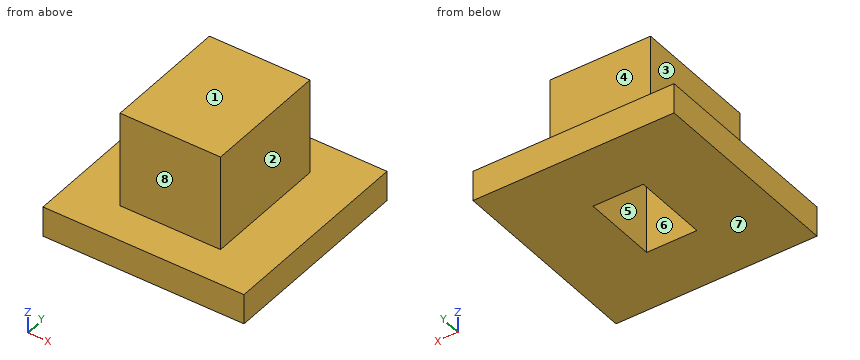
from build123d import *

# Parameters (mm, degrees)
SKETCH_1_W      = 4
SKETCH_1_H      = 5
SKETCH_1_W_2    = 2
SKETCH_1_H_2    = 3
EXTRUDE_1_DEPTH = 4
EXTRUDE_2_DEPTH = 1.2
SKETCH_3_W      = 4
SKETCH_3_H      = 5
EXTRUDE_3_DEPTH = 1
SKETCH_4_W      = 2
SKETCH_4_H      = 8
EXTRUDE_4_DEPTH = 1.2


with BuildPart() as part:
    # 草图1 → 凸台-拉伸1 (new body)
    with BuildSketch(Plane.XY):
        with Locations((1, 1.5)):
            Rectangle(SKETCH_1_W, SKETCH_1_H)
        with Locations((1, 1.5)):
            Rectangle(SKETCH_1_W_2, SKETCH_1_H_2, mode=Mode.SUBTRACT)
    extrude(amount=EXTRUDE_1_DEPTH)

    # 草图2 → 凸台-拉伸2 (add)
    with BuildSketch(Plane(origin=(0, 0, 0), x_dir=(-1, 0, 0), z_dir=(0, 0, -1))):
        Polygon((-3, 4), (1, 4), (1, -1), (-3, -1), (-3, -2.5), (3, -2.5), (3, 5.5), (-3, 5.5), align=None)
    extrude(amount=-EXTRUDE_2_DEPTH)

    # 草图3 → 凸台-拉伸3 (add)
    with BuildSketch(Plane.XY.offset(4)):
        with Locations((1, 1.5)):
            Rectangle(SKETCH_3_W, SKETCH_3_H)
    extrude(amount=EXTRUDE_3_DEPTH)

    # 草图4 → 凸台-拉伸4 (add)
    with BuildSketch(Plane.XY.offset(1.2)):
        with Locations((4, 1.5)):
            Rectangle(SKETCH_4_W, SKETCH_4_H)
    extrude(amount=-EXTRUDE_4_DEPTH)


solid = part.part
CAD build for the part. Positions are in the model's coordinates, mm. Face numbers are marked on the shaded views. A direction names the side the tool comes from. Give positions to 0.01 mm unless a question says otherwise; leave off trailing zeros. Loops run counter-clockwise (first coordinate to the right, second up) from the corner with the lowest first, then second, coordinate; pieces in that order, holes last. Notation, with made-up numbers: M 30.25,76.25 L 85.25,76.25 A30 ccw 85.25,109.25 Z; hole C 87.5,-32.75 d5. An arc over 180 degrees is marked long. Answer in a Markdown table with one row per item. Add a question column.
Item 1: Mould opens along Y. For the marked faces 5, 6, 7 and 8 say: +Y half, -Y half, draft (parallel to the pull), parting line (faces both ways), or undercut.
Item 2: Band-saw the part on D-D on z = 2.8. Give the cut face in (x, y).
Item 3: Drop flat-ended pins along their axis: P1, Ø3, axis at x = -1, z = 4, coming from the +Y side; P2, Ø0.9, axis at y = 1.5, z = 2.5, coming from the -X side; P3, Ø1.9, axis at y = 1, z = 3, coming from the +X side. Give the stop position or say it passes through.
Item 4: Tool access for the marked faces 1, 2, 3 and 4: list every direction of +Z, -Z, +X, -X, +Y, -Y with a clear straight run to the whole face (end or side of a thin tool).
Item 5: Band-saw the part on B-B on y = -0.5. Give the cut face in (x, z).
Item 6: Band-saw the part on A-A on z = 0.8. Give the cut face in (x, y).
Item 7: Probe probe 1 along Y at (x, z) = (0.75, 1.05); probe 2 along X at (y, z) = (0.5, 3.1); probe 3 along Y at (x, z) = (1.25, 2.1). List the from-to ranges inside material, lowest first.
Item 8: Band-saw the part on C-C on x = -0.25. Give the cut face in (y, z), then the cut area to 3 significant figures.
Reply:
| question | item | result |
|---|---|---|
| 1 | face 5 | undercut |
| 1 | face 6 | undercut |
| 1 | face 7 | draft |
| 1 | face 8 | -Y half |
| 2 | outline | M -1,-1 L 3,-1 L 3,4 L -1,4 Z; hole M 0,0 L 2,0 L 2,3 L 0,3 Z |
| 3 | P1 | stops at y = 4 |
| 3 | P2 | stops at x = -1 |
| 3 | P3 | stops at x = 3 |
| 4 | face 1 | +Z, +X, -X, +Y, -Y |
| 4 | face 2 | +Z, +X, +Y, -Y |
| 4 | face 3 | +Z, -X, +Y, -Y |
| 4 | face 4 | +Z, +X, -X, +Y |
| 5 | outline | M -3,0 L 5,0 L 5,1.2 L 3,1.2 L 3,5 L -1,5 L -1,1.2 L -3,1.2 Z |
| 6 | outline | M -3,-2.5 L 5,-2.5 L 5,5.5 L -3,5.5 Z; hole M 0,0 L 2,0 L 2,3 L 0,3 Z |
| 7 | probe 1 | y = -2.5 to 0, 3 to 5.5 |
| 7 | probe 2 | x = -1 to 0, 2 to 3 |
| 7 | probe 3 | y = -1 to 0, 3 to 4 |
| 8 | outline | M -2.5,0 L 5.5,0 L 5.5,1.2 L 4,1.2 L 4,5 L -1,5 L -1,1.2 L -2.5,1.2 Z |
| 8 | area | 28.6 mm^2 |
